Autodesk Inventor part; units mm, degrees
ref_plane "YZ Plane" through (0, 0, 0) normal (1, 0, 0) x (0, 1, 0)
ref_plane "XZ Plane" through (0, 0, 0) normal (0, 1, 0) x (-1, 0, 0)
ref_plane "XY Plane" through (0, 0, 0) normal (0, 0, 1) x (1, 0, 0)
sketch "Sketch1" plane through (0, 0, 0) normal (0, 0, 1) x (1, 0, 0)
  line L0 (0, 0) -> (-111.3151, 0)
  line L1 (-111.3151, 0) -> (-111.3151, -1489.5)
  line L2 (-111.3151, -1489.5) -> (0, -1489.5)
  line L3 (0, -1489.5) -> (0, 0)
  line L4 (-111.3151, -1389.5) -> (-66, -1389.5)
  line L5 (-66, -1389.5) -> (-66, -1384.5)
  line L6 (-66, -1384.5) -> (-111.3151, -1384.5)
  line L7 (-111.3151, -1384.5) -> (-111.3151, -1389.5)
  line L8 (-111.3151, -893) -> (-66, -893)
  line L9 (-66, -893) -> (-66, -888)
  line L10 (-66, -888) -> (-111.3151, -888)
  line L11 (-111.3151, -888) -> (-111.3151, -893)
  line L12 (-111.3151, -396.5) -> (-66, -396.5)
  line L13 (-66, -396.5) -> (-66, -391.5)
  line L14 (-66, -391.5) -> (-111.3151, -391.5)
  line L15 (-111.3151, -391.5) -> (-111.3151, -396.5)
  circle A0 centre (-111.3151, -154.5) radius 30
  point P0 (-111.3151, -391.5)
  point P1 (-111.3151, -1384.5)
  point P2 (-111.3151, -124.5)
  point P3 (-111.3151, -184.5)
  dimension "d0" = 1489.5
  dimension "d1" = 111.3151
  dimension "d2" = 5
  dimension "d4" = 100
  dimension "d7" = 496.5
  dimension "d23" = 66
  dimension "d28" = 60
  dimension "d29" = 1335
extrude "Plate1" add sketch "Sketch1" along normal blind 4 contours L3 L2 L1 L4 L5 L6 L8 L9 L10 L12 L13 L14 A0 L0
sketch "Sketch2" plane through (-4, 0, 0) normal (1, 0, 0) x (0, 1, 0)
  line L0 (-1489.5, 0) -> (0, 0)
  line L1 (0, 0) -> (0, 60)
  line L2 (0, 60) -> (-1489.5, 60)
  line L3 (-1489.5, 60) -> (-1489.5, 0)
edge flange "Flange1" height 60 angle 90 thickness 4 bend radius 4 thickness toward (1, 0, 0) relief tear relief width 4 relief depth 2 edges at (0, -744.75, 4) wall of the first edge with corners at (-4, -1489.5, 0) (-4, 0, 0) (-4, 0, 60) (-4, -1489.5, 60)
bend "Bend1"
corner "Corner1"
chamfer "Corner Chamfer1" distance 3 angle 45 6 edges at (-111.3151, -1389.5, 2) (-111.3151, -1384.5, 2) (-111.3151, -893, 2) (-111.3151, -888, 2) (-111.3151, -391.5, 2) (-111.3151, -396.5, 2)
sketch "Sketch4" plane through (0, -1489.5, 60) normal (1, 0, 0) x (0, 0, -1)
  circle A0 centre (18, 1139.5) radius 9
  line L0 (0, 0) -> (0, 1489.5)
  circle A1 centre (18, 642.8333) radius 9
  circle A2 centre (18, 146.1667) radius 9
  point P0 (60, 1489.5)
  dimension "d30" = 18
  dimension "d31" = 18
  dimension "d32" = 350
  dimension "d35" = 496.6667
extrude "Cut1" cut sketch "Sketch4" against normal blind 4
equation "\"d0\" = Стрингер_длина"
equation "\"d1\" = стрингер_глубина_8"
equation "\"d2\" = паз_под_стрингер_толщина"
equation "\"d7\" = 0.333333 * Стрингер_длина"
equation "\"d23\" = паз_под_стрингер_глубина - Thickness"
equation "\"d28\" = 2 * радиус_выреза_под_сварку"
equation "\"d35\" = Шаг_шпангоутов"
equation "\"d40\" = Thickness"
equation "\"d12\" = Thickness"
equation "\"d13\" = BendReliefWidth"
equation "\"d14\" = BendReliefDepth"
equation "\"d15\" = MinimumRemnant"
equation "\"d16\" = TransitionRadius"
equation "\"d17\" = ребро_усилителей"
equation "\"d19\" = BendRadius"
equation "\"d20\" = CornerReliefSize"
equation "\"d21\" = GapSize"
equation "\"d22\" = JacobiRadiusSize"
equation "\"BendRadius\" = Thickness"
equation "\"BendReliefWidth\" = Thickness"
equation "\"BendReliefDepth\" = 0.5 * Thickness"
equation "\"CornerReliefSize\" = 4 * Thickness"
equation "\"MinimumRemnant\" = 2 * Thickness"
equation "\"TransitionRadius\" = BendRadius"
equation "\"JacobiRadiusSize\" = BendRadius"
equation "\"GapSize\" = Thickness"
properties part number "GBK 0303 stringer 8" material "Steel"
Input: part model. Units: mm. Frame: model coordinates. A direction names the side the tool comes from. Give positions to 0.01 mm unless a question says otherwise; leave off trailing zeros. Order: outer loops, then holes, each group sorted by start corner. A loop starts at its lowest first (then second) coordinate and runs counter-clockwise, first axis right, second up. Notation, with made-up numbers: (41, 54) -> (54, 54) arc R14 ccw to (54, 74) -> close; hole circle Ø4 at (80, 45). An arc over 180 degrees is marked (long way). Use one line per item in the form item = value.
1) Reachability of faces 5 (the flat face through (-60, -734, 4)), 6 (the flat face through (-60, -734, 0)) from +Z, -Z, +X, -X, +Y, -Y: full face, straight path, thin tool, end or side. Return the list, or none.
Response values:
face_5 = +Z, -X, +Y, -Y
face_6 = -Z, +X, -X, +Y, -Y
2) Line query: probe 1 along Y at (x, z) = (-2.8, 42); probe 2 along Z at (x, y) = (-96, -226.5); probe 3 along X at (y, z) = (-1354, 20.5). Output: solid intervals per line, ascending.
Response values:
probe_1 = -1489.5 to -1352.33, -1334.33 to -855.67, -837.67 to -359, -341 to 0
probe_2 = 0 to 4
probe_3 = -4 to 0
3) Section C-C, the plane x = -33. Return loops of the section in (y, z).
Response values:
outline = (-1489.5, 0) -> (0, 0) -> (0, 4) -> (-1489.5, 4) -> close
4) Section B-B, the plane y = -695.5. Return loops of the section in (x, z).
Response values:
outline = (-111.32, 0) -> (-8, 0) arc R8 ccw to (0, 8) -> (0, 60) -> (-4, 60) -> (-4, 8) arc R4 cw to (-8, 4) -> (-111.32, 4) -> close
5) Section A-A, the plane z = 42. Return loops of the section in (x, y).
Response values:
outline = (-4, -1489.5) -> (0, -1489.5) -> (0, -1352.33) -> (-4, -1352.33) -> close; (-4, -1334.33) -> (0, -1334.33) -> (0, -855.67) -> (-4, -855.67) -> close; (-4, -837.67) -> (0, -837.67) -> (0, -359) -> (-4, -359) -> close; (-4, -341) -> (0, -341) -> (0, 0) -> (-4, 0) -> close
6) First-contact query: pin 1 Ø4.5 at (y, z) = (-393, 2) entering from -X; pin 2 Ø3 at (y, z) = (-1199, 21.5) entering from +X; pin 3 Ø3 at (y, z) = (-890.5, 1.5) entering from -X; pin 4 Ø4.5 at (y, z) = (-1387.5, 2.5) entering from -X. Flat tips, straight axial feed; report the tip coordinate or a pass-through.
Response values:
pin_1 = -109.07
pin_2 = 0
pin_3 = -66
pin_4 = -108.57
7) Mould query, pull axis Y, two halves, no side actions, for faces 1 (the cylindrical face through (-81.322, -153.84, 1.972)), 2 (the flat face through (-39, 0, 3)), 3 (the flat face through (0, -734, 34)), 4 (the flat face through (-39, -1489.5, 3)). Classes: pulls with the +Y half, pulls with the -Y half, needs draft (parallel to the pull), parting line crosses it, or undercut.
Response values:
face_1 = undercut
face_2 = pulls with the +Y half
face_3 = needs draft
face_4 = pulls with the -Y half
8) Section D-D, the plane y = -154.5. Return loops of the section in (x, z).
Response values:
outline = (-81.32, 0) -> (-8, 0) arc R8 ccw to (0, 8) -> (0, 60) -> (-4, 60) -> (-4, 8) arc R4 cw to (-8, 4) -> (-81.32, 4) -> close
